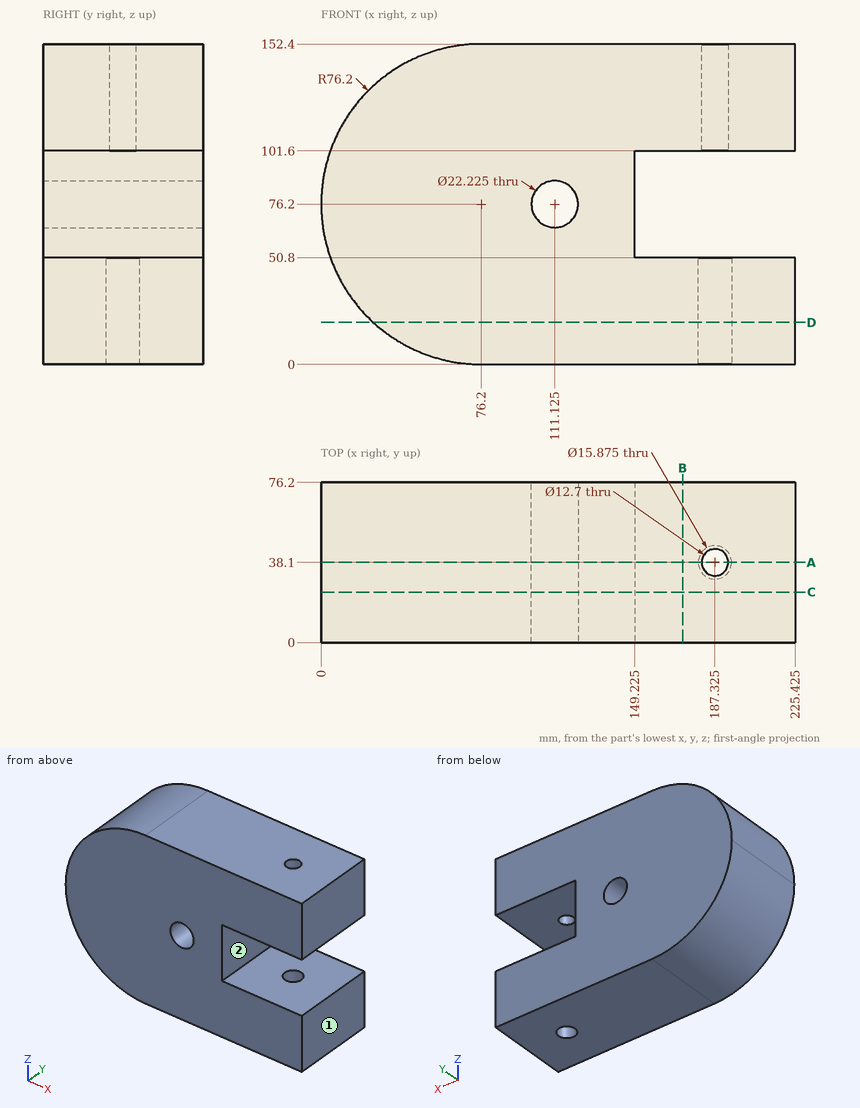
The drawing under review shows one solid part. Ordinate dimensions are in mm from its lowest x, y, z. A direction names the side the tool comes from. Round coordinates to 2 decimals unless told otherwise and drop trailing zeros. Write each loop counter-clockwise with the first axis right and the second up, starting at its lowest first coordinate (ties: lowest second). Pieces come first, ordered by that corner, then holes.
(1) We need section B-B on x = 172. Give the boundary of the cut face in (y, z), and give its area (3 significant figures).
(2) We need section A-A on y = 38.1. Give the boundary of the cut face in (x, z) (1 decimal).
(3) Wall thickness on L1, parallel to Z at x = 162, y = 34; L2, parallel to X at y = 51, z = 76 (3 decimals); L3, parallel to Y at x = 188, z = 17.5: over which ranges is each line inside the solid? List them lowest first.
(4) Insertion check: pin 1 (10 mm diameter, centred on x = 23, z = 66.5, fed in from -Y); pin 2 (12 mm diameter, centred on y = 19, z = 68, fed in from -X); pin 3 (5 mm diameter, centred on y = 53, z = 15.5, fed in from -X); pin 4 (1 mm diameter, centred on y = 20, z = 97, fed in from +X) (3 decimals). Each pin has a flat end and moves straight along its axis. Give the tip position at first contact, or say it passes through.
(5) Machinability: for the marked faces 1 and 2, which of the approach directions +Z, -Z, +X, -X, +Y, -Y give a long, thin tool a straight path to every point of the face, cutting with its end or side? Answer none if there is none.
(6) We need section C-C on y = 24. Give the boundary of the cut face in (x, z) (1 decimal).
(7) We need section D-D on z = 20. Give the boundary of the cut face in (x, y) (1 decimal), and give its area (3 significant figures).
Findings below:
1. outline: (0, 0) - (76.2, 0) - (76.2, 50.8) - (0, 50.8) - close; (0, 101.6) - (76.2, 101.6) - (76.2, 152.4) - (0, 152.4) - close
1. area: 7,740 mm2
2. outline: (0, 76.2) arc R76.2 ccw to (76.2, 0) - (179.4, 0) - (179.4, 50.8) - (149.2, 50.8) - (149.2, 101.6) - (181, 101.6) - (181, 152.4) - (76.2, 152.4) arc R76.2 ccw to start; (193.7, 101.6) - (225.4, 101.6) - (225.4, 152.4) - (193.7, 152.4) - close; (195.3, 0) - (225.4, 0) - (225.4, 50.8) - (195.3, 50.8) - close; hole circle Ø22.2 at (111.1, 76.2)
3. L1: z = 0 to 50.8, 101.6 to 152.4
3. L2: x = 0 to 100.014, 122.236 to 149.225
3. L3: y = 0 to 30.19, 46.01 to 76.2
4. pin 1: stops at y = 0
4. pin 2: stops at x = 0.03
4. pin 3: stops at x = 27.01
4. pin 4: stops at x = 149.225
5. face 1: +Z, -Z, +X, +Y, -Y
5. face 2: +X, +Y, -Y
6. outline: (0, 76.2) arc R76.2 ccw to (76.2, 0) - (225.4, 0) - (225.4, 50.8) - (149.2, 50.8) - (149.2, 101.6) - (225.4, 101.6) - (225.4, 152.4) - (76.2, 152.4) arc R76.2 ccw to start; hole circle Ø22.2 at (111.1, 76.2)
7. outline: (24.7, 0) - (225.4, 0) - (225.4, 76.2) - (24.7, 76.2) - close; hole circle Ø15.9 at (187.3, 38.1)
7. area: 15,100 mm2
